Design review of the part built by this model. Coordinates are the model's own, in mm. Face numbers are marked on the shaded views. Coordinates: 2 decimals unless noted, no trailing zeros. Loops run counter-clockwise (first coordinate to the right, second up) from the corner with the lowest first, then second, coordinate; pieces in that order, holes last. Notation, with made-up numbers: (1.25, 20) -> (6.25, 20) arc R31 cw to (6.25, 54) -> close; hole circle Ø1 at (-7, 46). An arc over 180 degrees is marked (long way). Answer as a JSON object with one key per item and string values.
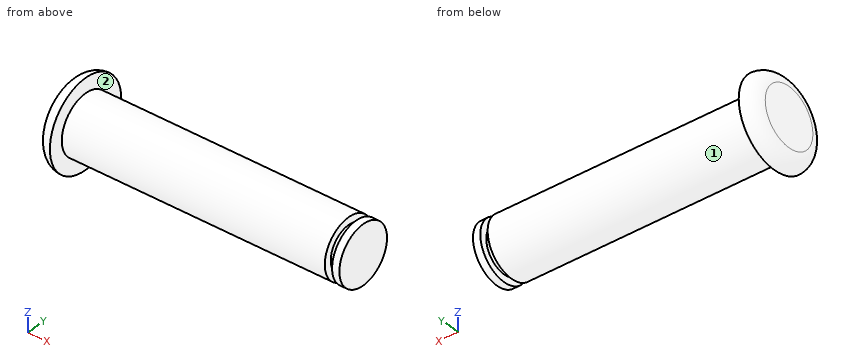
```python
from build123d import *


with BuildPart() as part:
    # Sketch1 → Revolve1 (revolve)
    with BuildSketch(Plane(origin=(0, 0, 0), x_dir=(-1, 0, 0), z_dir=(0, 0, -1))):
        with BuildLine():
            ThreePointArc((20, 2), (19.707106781, 2.707106781), (19, 3))
            Line((19, 3), (19, 2))
            Line((19, 2), (1, 2))
            Line((1, 2), (1, 1.5))
            Line((1, 1.5), (0.5, 1.5))
            Line((0.5, 1.5), (0.5, 2))
            Line((0.5, 2), (0, 2))
            Line((0, 2), (0, 0))
            Line((0, 0), (20, 0))
            Line((20, 0), (20, 2))
        make_face()
    revolve(axis=Axis((0, 0, 0), (-1, 0, 0)))


solid = part.part
```
1) Add section C-C, the plane x = -1.75. Give the boundary of the cut face in (y, z), and give its area (3 significant figures).
Completed:
{"outline": "circle Ø4 at (0, 0)", "area": "12.6 mm²"}
2) Add section A-A, the plane z = 0. Give the boundary of the cut face in (x, y).
Completed:
{"outline": "(-20, -2) arc R1 ccw to (-19, -3) -> (-19, -2) -> (-1, -2) -> (-1, -1.5) -> (-0.5, -1.5) -> (-0.5, -2) -> (0, -2) -> (0, 2) -> (-0.5, 2) -> (-0.5, 1.5) -> (-1, 1.5) -> (-1, 2) -> (-19, 2) -> (-19, 3) arc R1 ccw to (-20, 2) -> close"}
3) Wall thickness on probe 1 along X at (y, z) = (0.1, 1.8); probe 2 along Z at (x, y) = (-7.75, 1.8); probe 3 along Y at (x, z) = (-6.5, -1.75): over which ranges is each line inside the solid? List them lowest first.
Completed:
{"probe 1": "-20 to -1, -0.5 to 0", "probe 2": "-0.87 to 0.87", "probe 3": "-0.97 to 0.97"}
4) Clearance check with a flat-ended pin moving along its axis: pin 1 Ø1.5 at (x, y) = (-9, 1) entering from -Z. State where the tip first meets the part, or that it passes through.
Completed:
{"pin 1": "z = -1.98"}
5) The part is to be moulded in two halves that separate along Y. For the marked faces 1 and 2, say which applies: pulls with the +Y half, pulls with the -Y half, needs draft (parallel to the pull), parting line crosses it, or undercut.
Completed:
{"face 1": "parting line crosses it", "face 2": "needs draft"}
